from build123d import *


with BuildPart() as part:
    # Sketch → Revolve (revolve)
    with BuildSketch(Plane.XZ):
        with BuildLine():
            Line((18, 0), (18, 38.927282))
            ThreePointArc((18, 38.927282), (17.762487, 39.872608), (17.10636, 40.593406))
            Line((11.34046, 44.42215), (17.10636, 40.593406))
            ThreePointArc((10, 46.921335), (10.35627, 45.503347), (11.34046, 44.42215))
            Line((10, 73.35583), (10, 46.921335))
            ThreePointArc((10.852636, 74.993986), (10.225919, 74.279213), (10, 73.35583))
            Line((10.852636, 74.993986), (17.147364, 79.402814))
            ThreePointArc((17.147364, 79.402814), (17.774081, 80.117587), (18, 81.04097))
            Line((18, 81.04097), (18, 100))
            Line((18, 100), (16.5, 100))
            Line((16.5, 100), (16.5, 81.04097))
            ThreePointArc((15.647364, 79.402814), (16.274081, 80.117587), (16.5, 81.04097))
            Line((15.647364, 79.402814), (9.352636, 74.993986))
            ThreePointArc((9.352636, 74.993986), (8.725919, 74.279213), (8.5, 73.35583))
            Line((8.5, 73.35583), (8.5, 46.921335))
            ThreePointArc((8.5, 46.921335), (8.85627, 45.503347), (9.84046, 44.42215))
            Line((15.60636, 40.593406), (9.84046, 44.42215))
            ThreePointArc((16.5, 38.927282), (16.262487, 39.872608), (15.60636, 40.593406))
            Line((16.5, 0), (16.5, 38.927282))
            Line((18, 0), (16.5, 0))
        make_face()
    revolve(axis=Axis((0, 0, 0), (0, 0, 1)))


solid = part.part
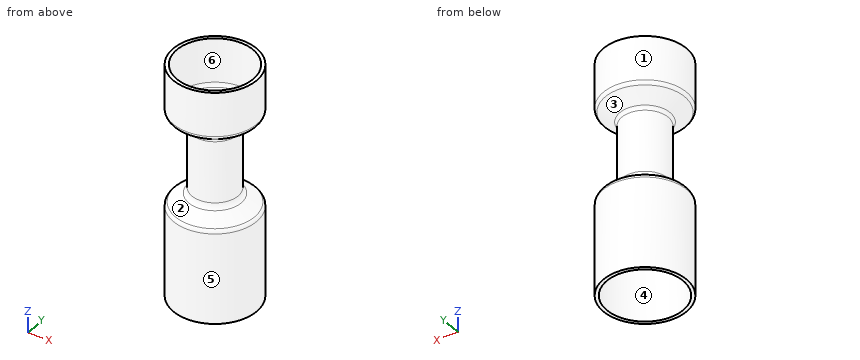
For this review, take the finished solid that the model builds, in its own axes (mm). Face numbers are marked on the shaded views. A direction names the side the tool comes from. Round coordinates to 2 decimals unless told otherwise and drop trailing zeros. Write each loop counter-clockwise with the first axis right and the second up, starting at its lowest first coordinate (ties: lowest second). Pieces come first, ordered by that corner, then holes. Notation, with made-up numbers: M 71,84.25 L 87,84.25 A16 cw 87,101.25 Z; hole C -26.75,-19 d2. An arc over 180 degrees is marked long. Write item = value, one per line. Start each with the question number.
(1) We need section B-B (z = 27). Give the boundary of the cut face in (x, y), then the cut area to 3 significant figures.
(2) Clearance check with flat-ended pins moving along their axes: pin 1 Ø15.5 at (x, y) = (0, 0) entering from -Z; pin 2 Ø5 at (x, y) = (11, 5) entering from -Z; pin 3 Ø6 at (y, z) = (-7.5, 15.5) entering from -X; pin 4 Ø3 at (x, z) = (-13.5, 28.5) entering from -Y. State where each tip first meets the part, or that it passes through.
(3) The part is to be moulded in two halves that separate along Z. For the marked faces 1 and 2, say which applies: +Z half, -Z half, draft (parallel to the pull), parting line (faces both ways), or undercut.
(4) For line 1 along Y through (x, z) = (0, 65.75); line 2 along Y through (x, z) = (-2, 72); line 3 along X through (y, z) = (-5.5, 40.5), list the stretches that pass through material, from the lowest coordinate up.
(5) We need section A-A (z = 55). Give the boundary of the cut face in (x, y), then the cut area to 3 significant figures.
(6) For the marked faces 3, 4, 5 and 6, list the 3-axis set-ups (+Z, -Z, +X, -X, +Y, -Y) from which the entire face can be reached by the end or side of a thin tool; tool diameter is ignored.
Results found:
q1.outline = C 0,0 d36; hole C 0,0 d33
q1.area = 163 mm²
q2.pin_1 = through
q2.pin_2 = 41.27
q2.pin_3 = -17.43
q2.pin_4 = -13.42
q3.face_1 = draft
q3.face_2 = undercut
q4.line_1 = -10 to -8.5, 8.5 to 10
q4.line_2 = -9.8 to -8.26, 8.26 to 9.8
q4.line_3 = -16.33 to -14.74, 14.74 to 16.33
q5.outline = C 0,0 d20; hole C 0,0 d17
q5.area = 87.2 mm²
q6.face_3 = none
q6.face_4 = -Z
q6.face_5 = +Z, -Z
q6.face_6 = +Z
